Model file for the job. Use its own axes, mm. A direction names the side the tool comes from. Coordinates: 2 decimals unless noted, no trailing zeros. Write each loop counter-clockwise with the first axis right and the second up, starting at its lowest first coordinate (ties: lowest second). Pieces come first, ordered by that corner, then holes. Notation, with made-up numbers: (61.5, 28) -> (80.5, 28) arc R14 cw to (80.5, 50) -> close; hole circle Ø9 at (89, 79.5). An arc over 180 degrees is marked (long way). Answer as a JSON object with one key per item and string values. Group by question number.
from build123d import *

# Parameters (mm, degrees)
BOSS_EXTRUDE1_DEPTH = 3.175


with BuildPart() as part:
    # Sketch1 → Boss-Extrude1 (new, symmetric)
    with BuildSketch(Plane(origin=(0, 0, 0), x_dir=(0, 0, -1), z_dir=(1, 0, 0))):
        Polygon((12.5, 23.075), (12.5, 13.55), (37.5, 13.55), (37.5, 0), (-37.5, 0), (-37.5, 13.55), (-12.5, 13.55), (-12.5, 23.075), align=None)
    boss_extrude1 = extrude(amount=BOSS_EXTRUDE1_DEPTH, both=True)

    # Mirror1: Boss-Extrude1 across plane
    add(boss_extrude1.mirror(Plane.ZX))


solid = part.part
(1) Pin check, flat tips, straight feed: pin 1 (3 mm diameter, centred on x = -0.5, y = -18, fed in from -Z); pin 2 (1.9 mm diameter, centred on x = 0, z = -25, fed in from -Y); pin 3 (2 mm diameter, centred on x = -1, z = 24.5, fed in from +Y). Stop position of each tip, or through.
(2) Cut at A-A on x = -1.5. List the corners of the cut face in (y, z) (3 decimals).
(3) Wall check: probe 1 along Z at (x, y) = (-0.5, 20); probe 2 along Y at (x, z) = (-1.75, -19). Give the ranges that are in metal, low to high.
(4) Cut at B-B on z = -25.5. List the corners of the cut face in (x, y) (3 decimals), plus the area to 3 significant figures.
(5) Cut at C-C on y = 16. List the corners of the cut face in (x, z) (3 decimals), plus the area to 3 significant figures.
(6) 3-axis set-ups, long thin cutter, end or side, ignore diameter. For faces 1 (the face through (0, -18, -12.5)), 2 (the face through (0, 18, -12.5)), 3 (the face through (0, 13.55, 25)): which of +Z, -Z, +X, -X, +Y, -Y reach the whole face in a straight line?
Results found:
{
 "1": {"pin 1": "stops at z = -12.5", "pin 2": "stops at y = -13.55", "pin 3": "stops at y = 13.55"},
 "2": {"outline": "(-23.075, -12.5) -> (-13.55, -12.5) -> (-13.55, -37.5) -> (13.55, -37.5) -> (13.55, -12.5) -> (23.075, -12.5) -> (23.075, 12.5) -> (13.55, 12.5) -> (13.55, 37.5) -> (-13.55, 37.5) -> (-13.55, 12.5) -> (-23.075, 12.5) -> close"},
 "3": {"probe 1": "z = -12.5 to 12.5", "probe 2": "y = -13.55 to 13.55"},
 "4": {"outline": "(-3.175, -13.55) -> (3.175, -13.55) -> (3.175, 13.55) -> (-3.175, 13.55) -> close", "area": "172 mm²"},
 "5": {"outline": "(-3.175, -12.5) -> (3.175, -12.5) -> (3.175, 12.5) -> (-3.175, 12.5) -> close", "area": "159 mm²"},
 "6": {"face 1": "-Z, +X, -X, -Y", "face 2": "-Z, +X, -X, +Y", "face 3": "+Z, +X, -X, +Y"}
}
